Work out the finished part from the listing and answer in its coordinate system (mm). Coordinates: 2 decimals unless noted, no trailing zeros. Order: outer loops, then holes, each group sorted by start corner. A loop starts at its lowest first (then second) coordinate and runs counter-clockwise, first axis right, second up. Notation, with made-up numbers: M 55.5,43.25 L 96.5,43.25 A27 cw 96.5,60.25 Z; hole C 43,-22.5 d8. An arc over 180 degrees is marked long. Answer in a Markdown table with one row per item. Add a question column.
Item 1: The part is cut by section C-C (z = 12.5). Write down the section's boundary in (x, y), then the cut area to 3 significant figures.
Item 2: The part is cut by section A-A (y = 0). Write down the section's boundary in (x, z), then the cut area to 3 significant figures.
Item 3: Consider line 1 (Y direction, x = 0, z = 7.75); line 2 (X direction, y = 8, z = 4.75); line 3 (Y direction, x = -6, z = 6.75). Determine where each line is inside the solid, lowest interval first. Write a range as from..to.
Item 4: The mould has two halves that part along X. Classify faces 1 (the face through (14, -14, 10)), 2 (the face through (-3.599, 16.205, 7.395)), 3 (the face through (8.767, -16.856, 4.93)): released by +X, released by -X, zero draft, split by the parting line, or undercut.
Item 5: Flat-ended cylindrical pins translate along their axes: pin 1 Ø1.5 at (x, y) = (-10.5, -15.5) entering from -Z; pin 2 Ø6 at (y, z) = (5, 12) entering from -X; pin 3 Ø12.5 at (x, y) = (-1, 6) entering from -Z; pin 4 Ø8 at (x, z) = (13, 4.5) entering from +Y. Find the tip coordinate at first contact, or state that the pin passes through.
Item 6: The part is cut by section D-D (z = 3.25). Write down the section's boundary in (x, y), then the cut area to 3 significant figures.
from build123d import *

# Parameters (mm, degrees)
F0_R     = 19
F1_DEPTH = 10
F2_R     = 20.5
F3_DEPTH = 5
F4_R     = 16.6
F5_DEPTH = 15.001


with BuildPart() as f1:
    # F0 (on Top) → F1 (new body)
    with BuildSketch(Plane.XY):
        Circle(F0_R)
    extrude(amount=F1_DEPTH)

    # F2 (on face) → F3 (join)
    with BuildSketch(Plane.XY.offset(10)):
        Circle(F2_R)
    extrude(amount=F3_DEPTH)

    # F4 (on face) → F5 (cut, through all)
    with BuildSketch(Plane(origin=(0, 0, 0), x_dir=(1, 0, 0), z_dir=(0, 0, -1))):
        Circle(F4_R)
    extrude(amount=-F5_DEPTH, mode=Mode.SUBTRACT)


solid = f1.part
Reply:
| question | item | result |
|---|---|---|
| 1 | outline | C 0,0 d41; hole C 0,0 d33.2 |
| 1 | area | 455 mm2 |
| 2 | outline | M -20.5,10 L -19,10 L -19,0 L -16.6,0 L -16.6,15 L -20.5,15 Z; M 16.6,0 L 19,0 L 19,10 L 20.5,10 L 20.5,15 L 16.6,15 Z |
| 2 | area | 87.0 mm2 |
| 3 | line 1 | y = -19..-16.6, 16.6..19 |
| 3 | line 2 | x = -17.23..-14.55, 14.55..17.23 |
| 3 | line 3 | y = -18.03..-15.48, 15.48..18.03 |
| 4 | face 1 | zero draft |
| 4 | face 2 | undercut |
| 4 | face 3 | split by the parting line |
| 5 | pin 1 | stops at z = 0 |
| 5 | pin 2 | stops at x = -20.4 |
| 5 | pin 3 | passes through |
| 5 | pin 4 | stops at y = 16.73 |
| 6 | outline | C 0,0 d38; hole C 0,0 d33.2 |
| 6 | area | 268 mm2 |
